Verification items for the finished model (mm, model axes). A direction names the side the tool comes from. Give positions to 0.01 mm unless a question says otherwise; leave off trailing zeros. Order: outer loops, then holes, each group sorted by start corner. A loop starts at its lowest first (then second) coordinate and runs counter-clockwise, first axis right, second up. Notation, with made-up numbers: (64.25, 64.5) - (116.25, 64.5) arc R8 cw to (116.25, 69.5) - close; hole circle Ø3 at (-37.75, 41.5). An arc over 180 degrees is marked (long way). Answer as a JSON object with one key per item and string values.
```python
from build123d import *

# Parameters (mm, degrees)
F0_R     = 49.609853
F1_DEPTH = 127
F2_R     = 10.853021
F3_DEPTH = 25.4
F4_R     = 12.7


with BuildPart() as f1:
    # F0 (on Top) → F1 (new body)
    with BuildSketch(Plane.XY):
        Circle(F0_R)
    extrude(amount=F1_DEPTH)

    # F2 (on face) → F3 (join)
    with BuildSketch(Plane.XY.offset(127)):
        Circle(F2_R)
    extrude(amount=F3_DEPTH)

    # F4
    f4_edges = [f1.edges().sort_by_distance(p)[0] for p in [
        (-49.609853, 0, 127),
        (49.609853, 0, 63.5),
        (-49.609853, 0, 0),
    ]]
    fillet(f4_edges, radius=F4_R)


solid = f1.part
```
(1) Gauge pin test, flat ends, axial feed: pin 1 Ø1 at (x, z) = (35.5, 27.5) entering from +Y; pin 2 Ø12 at (y, z) = (13.5, 23.5) entering from +X; pin 3 Ø2 at (y, z) = (-7.5, 21) entering from +X. Record the tip position at first contact, or that the pin passes through.
Computed values:
{"pin 1": "stops at y = 35.16", "pin 2": "stops at x = 49.04", "pin 3": "stops at x = 49.18"}
(2) Access from +Z, -Z, +X, -X, +Y, -Y to the whole of each face (thin tool, end or side, straight path). Record for faces 1 (the cylindrical face through (-10.843, 0.477, 139.522)), 2 (the cylindrical face through (-10.75, -48.43, 62.79)).
Computed values:
{"face 1": "+Z", "face 2": "+Z, -Z"}
(3) Material ranges on line 1 along Y through (x, z) = (0, 24); line 2 along Z through (x, y) = (21, -15); line 3 along Y through (x, z) = (-3, 123), recorded low to high. Write a range as [from, to].
Computed values:
{"line 1": "y = [-49.61, 49.61]", "line 2": "z = [0, 127]", "line 3": "y = [-46.06, 46.06]"}
(4) Section check A-A (y = 0). Record the cut outline in (x, z), then the cut area to 3 significant figures.
Computed values:
{"outline": "(-49.61, 12.7) arc R12.7 ccw to (-36.91, 0) - (36.91, 0) arc R12.7 ccw to (49.61, 12.7) - (49.61, 114.3) arc R12.7 ccw to (36.91, 127) - (10.85, 127) - (10.85, 152.4) - (-10.85, 152.4) - (-10.85, 127) - (-36.91, 127) arc R12.7 ccw to (-49.61, 114.3) - close", "area": "13,000 mm²"}
(5) Section check D-D (z = 120.5). Record the cut outline in (x, y), then the cut area to 3 significant figures.
Computed values:
{"outline": "circle Ø95.99 at (0, 0)", "area": "7,240 mm²"}
(6) Section check C-C (z = 55.5). Record the cut outline in (x, y), then the cut area to 3 significant figures.
Computed values:
{"outline": "circle Ø99.22 at (0, 0)", "area": "7,730 mm²"}
